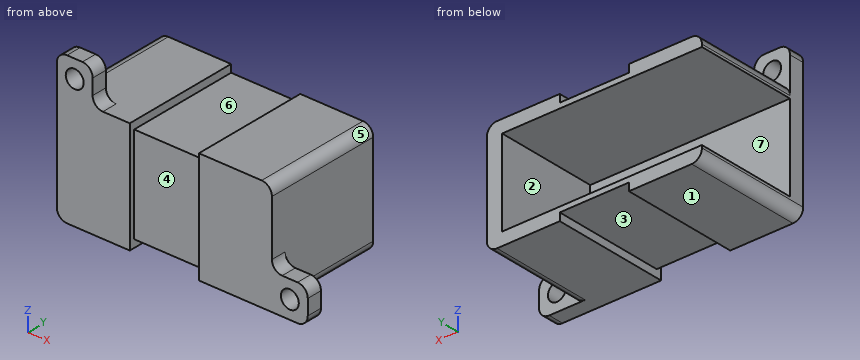
```python
from build123d import *

# Parameters (mm, degrees)
SKETCH1_W               = 3.5
SKETCH1_H               = 1
SKETCH1_H_2             = 1.5
SKETCH1_W_2             = 13.5
SKETCH1_W_3             = 11.25
SKETCH1_H_3             = 16.8
BOSS_EXTRUDE1_DEPTH     = 3
BOSS_EXTRUDE2_START     = 3
SKETCH1_5_W             = 3.5
SKETCH1_5_H             = 1
SKETCH1_5_H_2           = 1.5
SKETCH1_5_W_2           = 13.5
BOSS_EXTRUDE2_DEPTH     = 20
SKETCH1_7_W             = 13.5
SKETCH1_7_H             = 1.5
CUT_EXTRUDE1_DEPTH      = 24
CUT_EXTRUDE1_DEPTH_BACK = 1
SKETCH1_8_W             = 13.5
SKETCH1_8_H             = 16.8
SKETCH1_8_H_2           = 1.5
SKETCH1_8_H_3           = 1
CUT_EXTRUDE2_DEPTH      = 1
SKETCH2_W               = 7
SKETCH2_H               = 7
SKETCH2_R               = 1.75
BOSS_EXTRUDE3_DEPTH     = 3
FILLET1_R               = 2


with BuildPart() as part:
    # Sketch1 → Boss-Extrude1 (new body)
    with BuildSketch(Plane(origin=(0, 0, 0), x_dir=(1, 0, 0), z_dir=(0, 1, 0))):
        Polygon((-5.5, 11.1), (5.25, 11.1), (5.25, 27.9), (-9, 27.9), (-9, 11.1), align=None)
        Polygon((-9, 27.9), (5.25, 27.9), (5.25, 28.9), (5.25, 30.4), (-2, 30.4), (-9, 30.4), align=None)
        Polygon((-5.5, 8.6), (5.25, 8.6), (5.25, 10.1), (5.25, 11.1), (-5.5, 11.1), (-5.5, 9.6), align=None)
        with Locations((-7.25, 9.1)):
            Rectangle(SKETCH1_W, SKETCH1_H)
        with Locations((-7.25, 10.35)):
            Rectangle(SKETCH1_W, SKETCH1_H_2)
        with Locations((12, 10.6)):
            Rectangle(SKETCH1_W_2, SKETCH1_H)
        with Locations((12, 9.35)):
            Rectangle(SKETCH1_W_2, SKETCH1_H_2)
        Polygon((18.75, 10.1), (18.75, 8.6), (30, 8.6), (33, 8.6), (33, 11.1), (30, 11.1), (18.75, 11.1), align=None)
        Polygon((30, 11.1), (33, 11.1), (33, 30.4), (18.75, 30.4), (18.75, 28.9), (18.75, 27.9), (30, 27.9), align=None)
        with Locations((12, 28.4)):
            Rectangle(SKETCH1_W_2, SKETCH1_H)
        with Locations((12, 29.65)):
            Rectangle(SKETCH1_W_2, SKETCH1_H_2)
        with Locations((24.375, 19.5)):
            Rectangle(SKETCH1_W_3, SKETCH1_H_3)
        with Locations((12, 19.5)):
            Rectangle(SKETCH1_W_2, SKETCH1_H_3)
    extrude(amount=BOSS_EXTRUDE1_DEPTH)

    # Sketch1<5> → Boss-Extrude2 (add)
    with BuildSketch(Plane(origin=(0, 0, 0), x_dir=(1, 0, 0), z_dir=(0, 1, 0)).offset(BOSS_EXTRUDE2_START)):
        Polygon((-9, 27.9), (5.25, 27.9), (5.25, 28.9), (5.25, 30.4), (-2, 30.4), (-9, 30.4), align=None)
        Polygon((-5.5, 8.6), (5.25, 8.6), (5.25, 10.1), (5.25, 11.1), (-5.5, 11.1), (-5.5, 9.6), align=None)
        with Locations((-7.25, 9.1)):
            Rectangle(SKETCH1_5_W, SKETCH1_5_H)
        with Locations((-7.25, 10.35)):
            Rectangle(SKETCH1_5_W, SKETCH1_5_H_2)
        Polygon((18.75, 10.1), (18.75, 8.6), (30, 8.6), (33, 8.6), (33, 11.1), (30, 11.1), (18.75, 11.1), align=None)
        with Locations((12, 10.6)):
            Rectangle(SKETCH1_5_W_2, SKETCH1_5_H)
        Polygon((30, 11.1), (33, 11.1), (33, 30.4), (18.75, 30.4), (18.75, 28.9), (18.75, 27.9), (30, 27.9), align=None)
        with Locations((12, 28.4)):
            Rectangle(SKETCH1_5_W_2, SKETCH1_5_H)
    extrude(amount=BOSS_EXTRUDE2_DEPTH)

    # Sketch1<7> → Cut-Extrude1 (cut, two sides)
    with BuildSketch(Plane(origin=(0, 0, 0), x_dir=(1, 0, 0), z_dir=(0, 1, 0))) as cut_extrude1_sk:
        with Locations((12, 29.65)):
            Rectangle(SKETCH1_7_W, SKETCH1_7_H)
        with Locations((12, 9.35)):
            Rectangle(SKETCH1_7_W, SKETCH1_7_H)
    extrude(amount=CUT_EXTRUDE1_DEPTH, mode=Mode.SUBTRACT)
    extrude(cut_extrude1_sk.sketch, amount=-CUT_EXTRUDE1_DEPTH_BACK, mode=Mode.SUBTRACT)

    # Sketch1<8> → Cut-Extrude2 (cut)
    with BuildSketch(Plane(origin=(0, 0, 0), x_dir=(1, 0, 0), z_dir=(0, 1, 0))):
        with Locations((12, 19.5)):
            Rectangle(SKETCH1_8_W, SKETCH1_8_H)
        with Locations((12, 29.65)):
            Rectangle(SKETCH1_8_W, SKETCH1_8_H_2)
        with Locations((12, 28.4)):
            Rectangle(SKETCH1_8_W, SKETCH1_8_H_3)
        with Locations((12, 9.35)):
            Rectangle(SKETCH1_8_W, SKETCH1_8_H_2)
        with Locations((12, 10.6)):
            Rectangle(SKETCH1_8_W, SKETCH1_8_H_3)
    extrude(amount=CUT_EXTRUDE2_DEPTH, mode=Mode.SUBTRACT)

    # Sketch2 → Boss-Extrude3 (add)
    with BuildSketch(Plane(origin=(0, 0, 0), x_dir=(-1, 0, 0), z_dir=(0, 1, 0))):
        with Locations((5.5, -5.1)):
            Rectangle(SKETCH2_W, SKETCH2_H)
        with Locations((5.5, -5.1)):
            Circle(SKETCH2_R, mode=Mode.SUBTRACT)
        with Locations((-36.5, -26.9)):
            Rectangle(SKETCH2_W, SKETCH2_H)
        with Locations((-36.5, -26.9)):
            Circle(SKETCH2_R, mode=Mode.SUBTRACT)
    extrude(amount=BOSS_EXTRUDE3_DEPTH)

    # Fillet1
    fillet1_edges = [part.edges().sort_by_distance(p)[0] for p in [
        (33, 11.5, -8.6),
        (-9, 13, -8.6),
        (-9, 11.5, -30.4),
        (33, 13, -30.4),
        (-9, 1.5, -1.6),
        (-2, 1.5, -1.6),
        (-2, 1.5, -8.6),
        (33, 1.5, -23.4),
        (40, 1.5, -23.4),
        (40, 1.5, -30.4),
    ]]
    fillet(fillet1_edges, radius=FILLET1_R)


solid = part.part
```
Check sheet for the modelled part. Datum: model origin and axes. Units: mm. Face numbers are marked on the shaded views. A direction names the side the tool comes from. Round coordinates to 2 decimals unless told otherwise and drop trailing zeros. Write each loop counter-clockwise with the first axis right and the second up, starting at its lowest first coordinate (ties: lowest second). Pieces come first, ordered by that corner, then holes. Notation, with made-up numbers: (8, 25) -> (20, 25) arc R29 ccw to (20, 55) -> close; hole circle Ø9 at (-17, 30.5). An arc over 180 degrees is marked (long way). Put each result on its own line as item: value.
(1) Mould release check, pull along X, two halves, no side actions. Record for the marked faces 4, 5, 6 and 7: released by +X, released by -X, zero draft, split by the parting line, or undercut.
Values found:
face 4: undercut
face 5: released by +X
face 6: undercut
face 7: zero draft
(2) Material ranges on line 1 (Z direction, x = -4.5, y = 9.5); line 2 (Z direction, x = 18.5, y = 15.75); line 3 (X direction, y = 10.5, z = -12), recorded low to high.
Values found:
line 1: z = -30.4 to -27.9, -11.1 to -8.6
line 2: z = -28.9 to -27.9, -11.1 to -10.1
line 3: x = 30 to 33
(3) Sectioned sample at D-D (x = 1.5). Enter the section's corners in (y, z), plus the area to 3 significant figures.
Values found:
outline: (0, -30.4) -> (23, -30.4) -> (23, -27.9) -> (3, -27.9) -> (3, -11.1) -> (23, -11.1) -> (23, -8.6) -> (0, -8.6) -> close
area: 165 mm^2
(4) Sectioned sample at C-C (y = 2). Enter the section's corners in (x, z), plus the area to 3 significant figures.
Values found:
outline: (-9, -28.4) arc R2 ccw to (-7, -30.4) -> (5.25, -30.4) -> (5.25, -28.9) -> (18.75, -28.9) -> (18.75, -30.4) -> (38, -30.4) arc R2 ccw to (40, -28.4) -> (40, -25.4) arc R2 ccw to (38, -23.4) -> (35, -23.4) arc R2 cw to (33, -21.4) -> (33, -10.6) arc R2 ccw to (31, -8.6) -> (18.75, -8.6) -> (18.75, -10.1) -> (5.25, -10.1) -> (5.25, -8.6) -> (0, -8.6) arc R2 cw to (-2, -6.6) -> (-2, -3.6) arc R2 ccw to (-4, -1.6) -> (-7, -1.6) arc R2 ccw to (-9, -3.6) -> close; hole circle Ø3.5 at (-5.5, -5.1); hole circle Ø3.5 at (36.5, -26.9)
area: 950 mm^2
(5) Tool access check on the marked faces 1, 2 and 3. Record the directions out of +Z, -Z, +X, -X, +Y, -Y that give a thin tool (end or side, any length) a straight path to the whole face; none if there is none.
Values found:
face 1: -Z, +X, -X, +Y, -Y
face 2: -X, +Y
face 3: -Z, +Y, -Y
(6) Sectioned sample at A-A (x = -5.5). Enter the section's corners in (y, z).
Values found:
outline: (0, -30.4) -> (23, -30.4) -> (23, -27.9) -> (3, -27.9) -> (3, -11.1) -> (23, -11.1) -> (23, -8.6) -> (3, -8.6) -> (3, -6.85) -> (0, -6.85) -> close; (0, -3.35) -> (3, -3.35) -> (3, -1.6) -> (0, -1.6) -> close
(7) Go/stop test with flat-tipped pins: pin 1 Ø1.5 at (x, y) = (31, 20) entering from +Z; pin 2 Ø10 at (x, y) = (16, 14.5) entering from -Z; pin 3 Ø8.5 at (y, z) = (14.5, -15.5) entering from -X; pin 4 Ø6.5 at (y, z) = (6.5, -18) entering from +X. Record where each tip stops, or that it passes through.
Values found:
pin 1: stops at z = -8.6
pin 2: stops at z = -30.4
pin 3: stops at x = 30
pin 4: stops at x = 33
(8) Sectioned sample at B-B (z = -5.1). Enter the section's corners in (x, y), plus the area to 3 significant figures.
Values found:
outline: (-9, 0) -> (-7.25, 0) -> (-7.25, 3) -> (-9, 3) -> close; (-3.75, 0) -> (-2, 0) -> (-2, 3) -> (-3.75, 3) -> close
area: 10.5 mm^2
